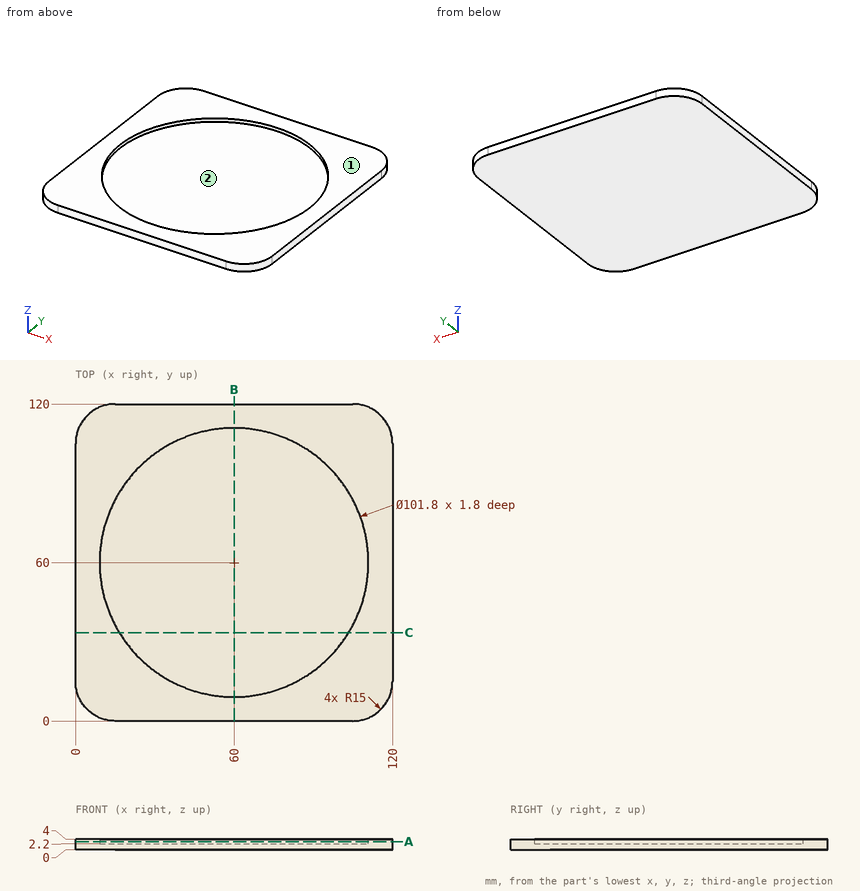
Part print with two shaded views. Sizes in mm from the minimum x, y, z corner. Coordinates: 2 decimals unless noted, no trailing zeros. Write each loop counter-clockwise with the first axis right and the second up, starting at its lowest first coordinate (ties: lowest second). Pieces come first, ordered by that corner, then holes. Notation, with made-up numbers: (26.25, 0) - (68.25, 0) arc R9 ccw to (68.25, 15) - close; hole circle Ø9 at (61, 50.5). An arc over 180 degrees is marked (long way). Use a Markdown table: item, result. Add a question column.
Item 1: Band-saw the part on B-B, the plane x = 60. Write the cut outline in (y, z), and give its area (3 significant figures).
Item 2: Drill centre lines: line 1 along X through (y, z) = (60, 3.3); line 2 along Z through (x, y) = (93.5, 47). Where is each one in solid material? Low to high.
Item 3: Two-plate mould, pull along Y, no slides. Class the marked faces 1 and 2: pulls with the +Y half, pulls with the -Y half, needs draft (parallel to the pull), parting line crosses it, or undercut.
Item 4: Band-saw the part on C-C, the plane y = 33.5. Write the cut outline in (x, z), and give its area (3 significant figures).
Item 5: Band-saw the part on A-A, the plane z = 3. Write the cut outline in (x, y), and give its area (3 significant figures).
Item 6: Drop a flat-ended pin along its axis: pin 1 (2 mm diameter, centred on x = 70, y = 107, fed in from +Z). Give the stop position or say it passes through.
A:
| question | item | result |
|---|---|---|
| 1 | outline | (0, 0) - (120, 0) - (120, 4) - (110.9, 4) - (110.9, 2.2) - (9.1, 2.2) - (9.1, 4) - (0, 4) - close |
| 1 | area | 297 mm² |
| 2 | line 1 | x = 0 to 9.1, 110.9 to 120 |
| 2 | line 2 | z = 0 to 2.2 |
| 3 | face 1 | needs draft |
| 3 | face 2 | undercut |
| 4 | outline | (0, 0) - (120, 0) - (120, 4) - (103.46, 4) - (103.46, 2.2) - (16.54, 2.2) - (16.54, 4) - (0, 4) - close |
| 4 | area | 324 mm² |
| 5 | outline | (0, 15) arc R15 ccw to (15, 0) - (105, 0) arc R15 ccw to (120, 15) - (120, 105) arc R15 ccw to (105, 120) - (15, 120) arc R15 ccw to (0, 105) - close; hole circle Ø101.8 at (60, 60) |
| 5 | area | 6,070 mm² |
| 6 | pin 1 | stops at z = 2.2 |
